Autodesk Inventor part; units mm, degrees
ref_plane "YZ Plane" through (0, 0, 0) normal (1, 0, 0) x (0, 1, 0)
ref_plane "XZ Plane" through (0, 0, 0) normal (0, 1, 0) x (-1, 0, 0)
sketch "スケッチ1" plane through (0, 0, 0) normal (0, 0, 1) x (1, 0, 0)
  circle A0 centre (0, 0) radius 2.5
  line L0 (-10, 10) -> (10, 10) construction
  line L1 (10, 10) -> (10, -10) construction
  line L2 (10, -10) -> (-10, -10) construction
  line L3 (-10, -10) -> (-10, 10) construction
  line L4 (-3, 10) -> (-3, 8.4) construction
  line L5 (-3, 8.4) -> (-6, 8.4) construction
  line L6 (-6, 8.4) -> (-6, 7.0607) construction
  line L7 (-6, 7.0607) -> (-3.3393, 4.4) construction
  line L8 (-3.3393, 4.4) -> (3.3393, 4.4) construction
  line L9 (3.3393, 4.4) -> (6, 7.0607) construction
  line L10 (6, 7.0607) -> (6, 8.4) construction
  line L11 (6, 8.4) -> (3, 8.4) construction
  line L12 (3, 8.4) -> (3, 10) construction
  line L13 (-10, 10) -> (10, -10) construction
  line L14 (-10, 10) -> (-3, 10)
  line L15 (-3, 10) -> (-3, 8.4)
  line L16 (-3, 8.4) -> (-6, 8.4)
  line L17 (-6, 8.4) -> (-6, 7.0607)
  line L18 (-6, 7.0607) -> (-3.3393, 4.4)
  line L19 (-3.3393, 4.4) -> (3.3393, 4.4)
  line L20 (3.3393, 4.4) -> (6, 7.0607)
  line L21 (6, 7.0607) -> (6, 8.4)
  line L22 (6, 8.4) -> (3, 8.4)
  line L23 (3, 8.4) -> (3, 10)
  line L24 (3, 10) -> (10, 10)
  line L25 (-10, -10) -> (-10, -3)
  line L26 (-10, -3) -> (-8.4, -3)
  line L27 (-8.4, -3) -> (-8.4, -6)
  line L28 (-8.4, -6) -> (-7.0607, -6)
  line L29 (-7.0607, -6) -> (-4.4, -3.3393)
  line L30 (-4.4, -3.3393) -> (-4.4, 3.3393)
  line L31 (-4.4, 3.3393) -> (-7.0607, 6)
  line L32 (-8.4, 6) -> (-8.4, 3)
  line L33 (-7.0607, 6) -> (-8.4, 6)
  line L34 (-8.4, 3) -> (-10, 3)
  line L35 (-10, 3) -> (-10, 10)
  line L36 (10, -10) -> (3, -10)
  line L37 (3, -10) -> (3, -8.4)
  line L38 (3, -8.4) -> (6, -8.4)
  line L39 (6, -8.4) -> (6, -7.0607)
  line L40 (6, -7.0607) -> (3.3393, -4.4)
  line L41 (3.3393, -4.4) -> (-3.3393, -4.4)
  line L42 (-3.3393, -4.4) -> (-6, -7.0607)
  line L43 (-6, -8.4) -> (-3, -8.4)
  line L44 (-6, -7.0607) -> (-6, -8.4)
  line L45 (-3, -8.4) -> (-3, -10)
  line L46 (-3, -10) -> (-10, -10)
  line L47 (10, 10) -> (10, 3)
  line L48 (10, 3) -> (8.4, 3)
  line L49 (8.4, 3) -> (8.4, 6)
  line L50 (8.4, 6) -> (7.0607, 6)
  line L51 (7.0607, 6) -> (4.4, 3.3393)
  line L52 (4.4, 3.3393) -> (4.4, -3.3393)
  line L53 (4.4, -3.3393) -> (7.0607, -6)
  line L54 (8.4, -6) -> (8.4, -3)
  line L55 (7.0607, -6) -> (8.4, -6)
  line L56 (8.4, -3) -> (10, -3)
  line L57 (10, -3) -> (10, -10)
  point P0 (-10, 0)
  point P1 (0, 10)
  dimension "d0" = 20
  dimension "d1" = 20
  dimension "d2" = 6
  dimension "d3" = 3
  dimension "d4" = 1.6
  dimension "d5" = 4
  dimension "d6" = 12
  dimension "d7" = 6
  dimension "d8" = 135
  dimension "d9" = 135
  dimension "d10" = 0.75
  dimension "d11" = 5
  dimension "d14" = 360
extrude "押し出し1" add sketch "スケッチ1" along normal mid plane 320
equation "\"d9\" = d8"
properties part number "l320"
Work out the finished part from the listing and answer in its coordinate system (mm). Coordinates: 2 decimals unless noted, no trailing zeros. Use one line per item in the form item = value. Start each with the question number.
1. The mould has two halves that part along Y. Classify faces 1 (the face through (-0.54, 2.44, -2.24)), 2 (the face through (2, -2, -160)), 3 (the face through (-6, -10, -2)): released by +Y, released by -Y, zero draft, split by the parting line, or undercut.
2. Straight lines are drawn through the part: probe 1 along Y at (x, z) = (0, 56.5); probe 2 along Y at (x, z) = (9, -111); probe 3 along X at (y, z) = (4.75, -18.5). For each, find the intervals that lie inside material, in ascending order. Write a range as from..to.
3. Each of these flat-tipped pins is pushed along its axis until it touches: P1, Ø2, axis at x = 0, z = -62.5, coming from the -Y side; P2, Ø1.5, axis at x = 0, z = -65, coming from the +Y side. Where does it stop, or does it pass through?
Evaluation:
q1.face_1 = undercut
q1.face_2 = zero draft
q1.face_3 = released by -Y
q2.probe_1 = -4.4..-2.5, 2.5..4.4
q2.probe_2 = -10..-3, 3..10
q2.probe_3 = -10..-8.4, -5.81..-3.69, 3.69..5.81, 8.4..10
q3.P1 = -4.4
q3.P2 = 4.4
